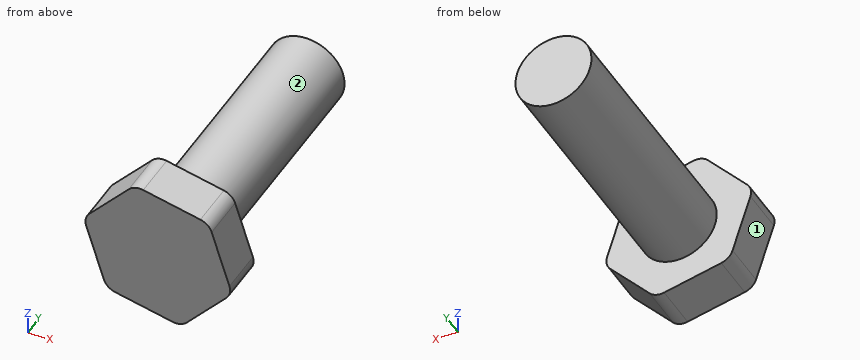
from build123d import *

# Parameters (mm, degrees)
EXTRUDE_1_DEPTH = 3
SKETCH_4_R      = 2.5
EXTRUDE_2_DEPTH = 16
FILLET_1_R      = 1


with BuildPart() as part:
    # 草图2 → 凸台-拉伸1 (new body)
    with BuildSketch(Plane(origin=(0, 0, 0), x_dir=(1, 0, 0), z_dir=(0, 1, 0))):
        Polygon((7.324934491, 4.171243509), (8.84728701, 8.933852332), (5.48392304, 12.633552699), (0.598206551, 11.570644242), (-0.924145968, 6.808035419), (2.439218002, 3.108335052), align=None)
    extrude(amount=EXTRUDE_1_DEPTH)

    # 草图4 → 凸台-拉伸2 (add)
    with BuildSketch(Plane(origin=(0, 3, 0), x_dir=(1, 0, 0), z_dir=(0, 1, 0))):
        with Locations(Location((3.961570521, 7.870943875, 0), (0, 0, 270))):
            Circle(SKETCH_4_R)
    extrude(amount=EXTRUDE_2_DEPTH)

    # 圆角1
    fillet_1_edges = [part.edges().sort_by_distance(p)[0] for p in [
        (8.84728701, 1.5, -8.933852332),
        (7.324934491, 1.5, -4.171243509),
        (2.439218002, 1.5, -3.108335052),
        (-0.924145968, 1.5, -6.808035419),
        (0.598206551, 1.5, -11.570644242),
        (5.48392304, 1.5, -12.633552699),
    ]]
    fillet(fillet_1_edges, radius=FILLET_1_R)


solid = part.part
Can you work these out from the model? Positions are in its coordinate system, mm. Face numbers are marked on the shaded views. A direction names the side the tool comes from. Coordinates: 2 decimals unless noted, no trailing zeros. Loops run counter-clockwise (first coordinate to the right, second up) from the corner with the lowest first, then second, coordinate; pieces in that order, holes last. Notation, with made-up numbers: (17, 14.5) - (67, 14.5) arc R22 ccw to (67, 51.5) - close; hole circle Ø5 at (2, 38). An arc over 180 degrees is marked (long way). Put each result on its own line as item: value. Start each with the question number.
Item 1: Which directions (+Z, -Z, +X, -X, +Y, -Y) give clear straight access to the entire face, cutting with the end or side of a thin tool? Please do the marked faces 1 and 2.
Item 2: Suppose I cut it at D-D (z = -4.5). Please give me the cut outline in (x, y).
Item 3: For pin 1 (5 mm diameter, centred on x = 1.5, y = 12.5, fed in from +Z); pin 2 (2 mm diameter, centred on x = 6.5, z = -11, fed in from +Y); pin 3 (1 mm diameter, centred on x = 6, y = 4, fed in from -Z), each with a flat end and sliding along its axis, tell me the tip position at first contact or that it passes through.
Item 4: Suppose I cut it at B-B (z = -8). Please give me the cut outline in (x, y).
Item 5: If I drill on line 1 along Y through (x, z) = (4, -11); line 2 along Z through (x, y) = (1.5, 1.75); line 3 along Z through (x, y) = (4.5, 6.25), over which ranges is the centre line in solid material (lowest first)?
Item 6: Suppose I cut it at A-A (x = 2.5). Please give me the cut outline in (y, z).
Item 7: Suppose I cut it at C-C (y = 10.75). Please give me the cut outline in (x, z), and give its area (3 significant figures).
Here are the results:
1. face 1: -Z, -X, +Y, -Y
1. face 2: +Y
2. outline: (1.17, 0) - (7.4, 0) - (7.4, 3) - (1.17, 3) - close
3. pin 1: z = -5.37
3. pin 2: y = 3
3. pin 3: z = -9.84
4. outline: (-0.54, 0) - (8.55, 0) - (8.55, 3) - (6.46, 3) - (6.46, 19) - (1.46, 19) - (1.46, 3) - (-0.54, 3) - close
5. line 1: 0 to 3
5. line 2: -11.77 to -4.14
5. line 3: -10.31 to -5.43
6. outline: (0, -11.98) - (3, -11.98) - (3, -9.9) - (19, -9.9) - (19, -5.84) - (3, -5.84) - (3, -3.25) - (0, -3.25) - close
7. outline: circle Ø5 at (3.96, -7.87)
7. area: 19.6 mm²
